CAD build for the part. Positions are in the model's coordinates, mm. A direction names the side the tool comes from. Coordinates: 2 decimals unless noted, no trailing zeros. Loops run counter-clockwise (first coordinate to the right, second up) from the corner with the lowest first, then second, coordinate; pieces in that order, holes last. Notation, with made-up numbers: (72, -14) -> (110, -14) arc R25 ccw to (110, 24) -> close; hole circle Ø11 at (61.5, 4.25). An arc over 180 degrees is marked (long way). Write each question's results on one line, items separated by ' | '.
from build123d import *
from build123d import SkipClean  # not in build123d's __all__

# Parameters (mm, degrees)
F1_DEPTH = 16
F2_R     = 1.7
F3_DEPTH = 25


with BuildPart() as f1:
    # F0 (on Top) → F1 (new body)
    with BuildSketch(Plane.XY):
        with BuildLine():
            ThreePointArc((0, -1.6), (-1.6, 0), (0, 1.6))
            Line((0, 1.6), (0, 3))
            Line((0, 3), (-9.7, 3))
            Line((-9.7, 3), (-9.7, 0))
            Line((-9.7, 0), (-9.7, -3))
            Line((-9.7, -3), (0, -3))
            Line((0, -3), (0, -1.6))
        make_face()
        Polygon((-8.2, -1.35), (-8.2, 0), (-8.2, 1.35), (-2.4, 1.35), (-2.4, -1.35), align=None, mode=Mode.SUBTRACT)
    extrude(amount=F1_DEPTH)

    # F2 (on face) → F3 (cut)
    with BuildSketch(Plane(origin=(0, 3, 0), x_dir=(-1, 0, 0), z_dir=(0, 1, 0))):
        with Locations((5.3, 13)):
            Circle(F2_R)
    extrude(amount=-F3_DEPTH, mode=Mode.SUBTRACT)

    # F4: F1 across plane


with BuildPart() as f1_1:
    add(f1.part, clean=False)
    with SkipClean():  # cleaning this boolean's faces spoils the solid; the shape is the same uncleaned
        add(f1.part.mirror(Plane.YZ), clean=False)


solid = f1_1.part
1) Slice it at C-C (y = 0). Write the cut outline in (x, z).
Outcome:
outline: (-9.7, 0) -> (-8.2, 0) -> (-8.2, 16) -> (-9.7, 16) -> close; (-2.4, 0) -> (-1.6, 0) -> (-1.6, 16) -> (-2.4, 16) -> close; (1.6, 0) -> (2.4, 0) -> (2.4, 16) -> (1.6, 16) -> close; (8.2, 0) -> (9.7, 0) -> (9.7, 16) -> (8.2, 16) -> close
2) Slice it at B-B (z = 13). Count the separate pieces of the cut face and the enclosed holes in it, then the cut area to 3 significant figures.
Outcome:
separate pieces: 3 | enclosed holes: 1 | area: 54.6 mm^2
3) Slice it at D-D (x = 2.75). Write the cut outline in (y, z), then the cut area to 3 significant figures.
Outcome:
outline: (-3, 0) -> (-1.35, 0) -> (-1.35, 16) -> (-3, 16) -> close; (1.35, 0) -> (3, 0) -> (3, 16) -> (1.35, 16) -> close | area: 52.8 mm^2
4) Which spindle directions (+Z, -Z, +X, -X, +Y, -Y) get a long thin tool onto all of the face, cutting with end or side? Do faces 4 (the flat face through (0, 2, 16)), 5 (the flat face through (-8.2, 0, 8)). Say none if no direction does.
Outcome:
face 4: +Z, +X, -X, +Y, -Y | face 5: +Z, -Z
5) Drill centre lines: L1, parallel to X at y = 0.05, z = 4.25; L2, parallel to Y at x = 2.75, z = 6.5; L3, parallel to X at y = -0.5, z = 9.75. Where is each one in solid material? Low to high. Write a range as from..to.
Outcome:
L1: x = -9.7..-8.2, -2.4..-1.6, 1.6..2.4, 8.2..9.7 | L2: y = -3..-1.35, 1.35..3 | L3: x = -9.7..-8.2, -2.4..-1.52, 1.52..2.4, 8.2..9.7
6) Two-plate mould, pull along X, no slides. Class faces 1 (the flat face through (0, -3, 8)), 2 (the flat face through (2.4, 0, 8)), 3 (the flat face through (-9.7, 0, 8)): pulls with the +X half, pulls with the -X half, needs draft (parallel to the pull), parting line crosses it, or undercut.
Outcome:
face 1: needs draft | face 2: undercut | face 3: pulls with the -X half
7) Slice it at A-A (x = 5.3). Write the cut outline in (y, z).
Outcome:
outline: (-3, 0) -> (-1.35, 0) -> (-1.35, 11.3) -> (-3, 11.3) -> close; (-3, 14.7) -> (-1.35, 14.7) -> (-1.35, 16) -> (-3, 16) -> close; (1.35, 0) -> (3, 0) -> (3, 11.3) -> (1.35, 11.3) -> close; (1.35, 14.7) -> (3, 14.7) -> (3, 16) -> (1.35, 16) -> close
